Autodesk Inventor part; units mm, degrees
ref_plane "YZ Plane" through (0, 0, 0) normal (1, 0, 0) x (0, 1, 0)
ref_plane "XZ Plane" through (0, 0, 0) normal (0, 1, 0) x (-1, 0, 0)
ref_plane "XY Plane" through (0, 0, 0) normal (0, 0, 1) x (1, 0, 0)
sketch "Sketch1" plane through (0, 0, 0) normal (0, 0, 1) x (1, 0, 0)
  line L0 (-684.25, 0) -> (684.25, 0) construction
  arc A0 (684.25, 12.5) -> (684.25, -12.5) centre (684.25, 0) ccw construction
  arc A1 (-684.25, -12.5) -> (-684.25, 12.5) centre (-684.25, 0) ccw construction
  arc A2 (684.25, 14) -> (684.25, -14) centre (684.25, 0) ccw construction
  arc A3 (-684.25, -14) -> (-684.25, 14) centre (-684.25, 0) ccw construction
  line L1 (684.25, 14) -> (-684.25, 14)
  line L2 (-684.25, 12.5) -> (684.25, 12.5)
  line L3 (684.25, -12.5) -> (-684.25, -12.5)
  line L4 (-684.25, -14) -> (684.25, -14)
  arc A4 (684.25, -14) -> (684.25, 14) centre (684.25, 0) ccw
  arc A5 (684.25, -12.5) -> (684.25, 12.5) centre (684.25, 0) ccw
  arc A6 (-684.25, 14) -> (-684.25, -14) centre (-684.25, 0) ccw
  arc A7 (-684.25, 12.5) -> (-684.25, -12.5) centre (-684.25, 0) ccw
  point P0 (0, 0)
  point P1 (0, 0)
  dimension "d0" = 1368.5
  dimension "d1" = 25
  dimension "d5" = 14
extrude "Extrusion1" add sketch "Sketch1" along normal mid plane 6
properties part number "correia-gt2"
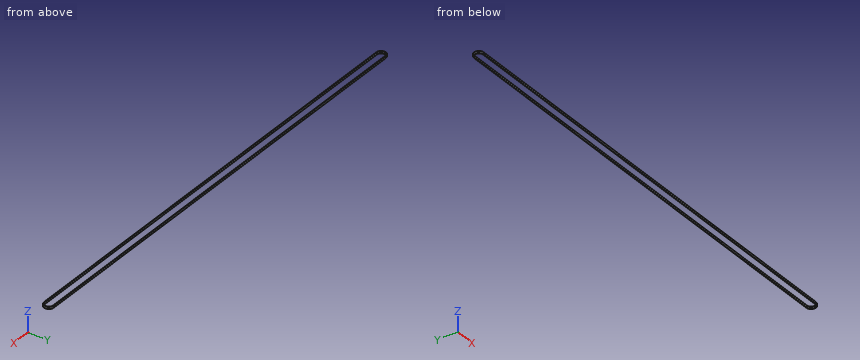
Design review of the part built by this model. Coordinates are the model's own, in mm. Give positions to 0.01 mm unless a question says otherwise; leave off trailing zeros. Loops run counter-clockwise (first coordinate to the right, second up) from the corner with the lowest first, then second, coordinate; pieces in that order, holes last. Notation, with made-up numbers: (-25, 54) - (-9, 54) arc R33 ccw to (-9, 83) - close; hole circle Ø9 at (85, 52). An arc over 180 degrees is marked (long way). Use CSV: the item, a comma, the result in double quotes. Start each with the question number.
1. Add section C-C (z = 1.85). State the section outline as (x, y) points, plus the area to 3 significant figures.
2. Add section B-B (y = 0). State the section outline as (x, z) points.
3. Wall thickness on L1, parallel to X at y = -1, z = 1.5; L2, parallel to Y at x = 561, z = 0.1; L3, parallel to X at y = -3, z = -1.6: over which ranges is each line inside the solid? List them lowest first.
4. Add section A-A (x = 472). State the section outline as (y, z) points, plus the area to 3 significant figures.
Results found:
1,outline,"(-684.25, -14) - (684.25, -14) arc R14 ccw to (684.25, 14) - (-684.25, 14) arc R14 ccw to start; hole (-684.25, -12.5) - (684.25, -12.5) arc R12.5 ccw to (684.25, 12.5) - (-684.25, 12.5) arc R12.5 ccw to start"
1,area,"4,230 mm²"
2,outline,"(-698.25, -3) - (-696.75, -3) - (-696.75, 3) - (-698.25, 3) - close; (696.75, -3) - (698.25, -3) - (698.25, 3) - (696.75, 3) - close"
3,L1,"x = -698.21 to -696.71, 696.71 to 698.21"
3,L2,"y = -14 to -12.5, 12.5 to 14"
3,L3,"x = -697.92 to -696.38, 696.38 to 697.92"
4,outline,"(-14, -3) - (-12.5, -3) - (-12.5, 3) - (-14, 3) - close; (12.5, -3) - (14, -3) - (14, 3) - (12.5, 3) - close"
4,area,"18.0 mm²"
